For this review, take the finished solid that the model builds, in its own axes (mm). Give positions to 0.01 mm unless a question says otherwise; leave off trailing zeros. Write each loop counter-clockwise with the first axis right and the second up, starting at its lowest first coordinate (ties: lowest second). Pieces come first, ordered by that corner, then holes. Notation, with made-up numbers: (20.25, 77.25) -> (47.25, 77.25) arc R10 ccw to (47.25, 86.25) -> close; hole circle Ø4 at (4, 3.25). An arc over 180 degrees is marked (long way). Answer as CSV lines item,"result".
```python
from build123d import *

# Parameters (mm, degrees)
F0_R     = 38.1
F1_DEPTH = 38.1
F3_D     = 10.0838


# Not quite as in the source:
# - a feature names something its author has since deleted; it is built from what else it names


with BuildPart() as f1:
    # F0 (on Front) → F1 (new body)
    with BuildSketch(Plane.XZ):
        with BuildLine():
            Line((0, 1358.9), (0, 0))
            Line((0, 0), (990.6, 0))
            Line((990.6, 0), (990.6, 241.3))
            Line((990.6, 241.3), (864.8059485884, 1247.6524112928))
            ThreePointArc((864.8059485884, 1247.6524112928), (822.8355837767, 1327.1091283286), (738.7866582458, 1358.9))
            Line((738.7866582458, 1358.9), (0, 1358.9))
        make_face()
        with Locations((787.4, 495.3)):
            Circle(F0_R, mode=Mode.SUBTRACT)
        with Locations((698.5, 1187.45)):
            Circle(F0_R, mode=Mode.SUBTRACT)
    extrude(amount=F1_DEPTH)

    # F3 (through all)
    with Locations(Plane.XZ.offset(38.1)):
        with Locations((82.55, 914.4), (127, 1066.8), (698.5, 1243.0125), (754.0625, 1187.45), (698.5, 1131.8875), (642.9375, 1187.45), (842.9625, 495.3), (787.4, 550.8625), (731.8375, 495.3), (787.4, 439.7375)):
            Hole(F3_D / 2)


solid = f1.part
```
Q1. Draft analysis for pull direction X (two halves, no side actions). For faces 1 (the flat face through (488, -19, 0)), 2 (the cylindrical face through (660.437, -18.783, 1189.125)), 3 (the cylindrical face through (823.8, -18.78, 1326.25)), state which applies: released by +X, released by -X, zero draft, split by the parting line, or undercut.
Answer block:
face 1,"zero draft"
face 2,"undercut"
face 3,"released by +X"
Q2. Add section D-D (z = 663). Write out the cut boundary in (x, y).
Answer block:
outline,"(0, -38.1) -> (937.89, -38.1) -> (937.89, 0) -> (0, 0) -> close"
Q3. Add section A-A (x = 808). Write out the cut boundary in (y, z).
Answer block:
outline,"(-38.1, 0) -> (0, 0) -> (0, 463.25) -> (-38.1, 463.25) -> close; (-38.1, 527.35) -> (0, 527.35) -> (0, 1338.38) -> (-38.1, 1338.38) -> close"
Q4. To check wall thickness, follow probe 1 along Z at (x, y) = (787.4, -26); probe 2 along Z at (x, y) = (787, -17); probe 3 along X at (y, z) = (-29, 1187). State the ranges of each line that lie inside material, in increasing order. Write a range as [from, to].
Answer block:
probe 1,"z = [0, 434.7], [444.78, 457.2], [533.4, 545.82], [555.9, 1349.23]"
probe 2,"z = [0, 434.71], [444.76, 457.2], [533.4, 545.84], [555.89, 1349.39]"
probe 3,"x = [0, 637.92], [647.96, 660.4], [736.6, 749.04], [759.08, 872.39]"
Q5. Clearance check with flat-ended pins moving along their axes: pin 1 (9 mm diameter, centred on x = 127, z = 1066.8, fed in from +Y); pin 2 (4 mm diameter, centred on x = 805, y = -6.5, fed in from +Z). State where each tip first meets the part, or that it passes through.
Answer block:
pin 1,"passes through"
pin 2,"stops at z = 1341.47"
Q6. Add section B-B (y = -10.5). State how many separate pieces and enclosed holes the cut face has, plus the area to 3 significant figures.
Answer block:
separate pieces,"1"
enclosed holes,"12"
area,"1,260,000 mm2"
Q7. Add section C-C (z = 837.5). Write out the cut boundary in (x, y) (3 decimals).
Answer block:
outline,"(0, -38.1) -> (916.075, -38.1) -> (916.075, 0) -> (0, 0) -> close"
